```python
from build123d import *

# Parameters (mm, degrees)
SALIENTE_EXTRUIR1_DEPTH = 3


with BuildPart() as part:
    # Model → Saliente-Extruir1 (new body)
    with BuildSketch(Plane.XY):
        with BuildLine():
            Line((149.34213351, 211.823953209), (158.34213351, 211.823953209))
            Line((158.34213351, 211.823953209), (162.84213351, 211.823953209))
            Line((162.84213351, 211.823953209), (162.84213351, 198.323953209))
            Line((162.84213351, 198.323953209), (162.84213351, 193.823953209))
            Line((162.84213351, 193.823953209), (158.34213351, 193.823953209))
            ThreePointArc((158.34213351, 193.823953209), (156.620058064, 194.166495313), (155.160152994, 195.141972694))
            Line((155.160152994, 195.141972694), (146.160152994, 204.141972694))
            ThreePointArc((146.160152994, 204.141972694), (145.184675613, 205.601877763), (144.84213351, 207.323953209))
            Line((144.84213351, 207.323953209), (144.84213351, 211.823953209))
            Line((144.84213351, 211.823953209), (149.34213351, 211.823953209))
        make_face()
        with BuildLine():
            Line((156.71713351, 195.823953209), (156.71713351, 200.823953209))
            ThreePointArc((156.71713351, 200.823953209), (156.936803424, 201.354283295), (157.46713351, 201.573953209))
            Line((157.46713351, 201.573953209), (159.21713351, 201.573953209))
            ThreePointArc((159.21713351, 201.573953209), (159.747463595, 201.354283295), (159.96713351, 200.823953209))
            Line((159.96713351, 200.823953209), (159.96713351, 195.823953209))
            ThreePointArc((159.96713351, 195.823953209), (159.747463595, 195.293623123), (159.21713351, 195.073953209))
            Line((159.21713351, 195.073953209), (157.46713351, 195.073953209))
            ThreePointArc((157.46713351, 195.073953209), (156.936803424, 195.293623123), (156.71713351, 195.823953209))
        make_face(mode=Mode.SUBTRACT)
        with BuildLine():
            Line((151.84213351, 205.698953209), (146.84213351, 205.698953209))
            ThreePointArc((146.84213351, 205.698953209), (146.311803424, 205.918623123), (146.09213351, 206.448953209))
            Line((146.09213351, 206.448953209), (146.09213351, 208.198953209))
            ThreePointArc((146.09213351, 208.198953209), (146.311803424, 208.729283295), (146.84213351, 208.948953209))
            Line((146.84213351, 208.948953209), (151.84213351, 208.948953209))
            ThreePointArc((151.84213351, 208.948953209), (152.372463595, 208.729283295), (152.59213351, 208.198953209))
            Line((152.59213351, 208.198953209), (152.59213351, 206.448953209))
            ThreePointArc((152.59213351, 206.448953209), (152.372463595, 205.918623123), (151.84213351, 205.698953209))
        make_face(mode=Mode.SUBTRACT)
        with BuildLine():
            Line((160.84213351, 205.698953209), (155.84213351, 205.698953209))
            ThreePointArc((155.84213351, 205.698953209), (155.311803424, 205.918623123), (155.09213351, 206.448953209))
            Line((155.09213351, 206.448953209), (155.09213351, 208.198953209))
            ThreePointArc((155.09213351, 208.198953209), (155.311803424, 208.729283295), (155.84213351, 208.948953209))
            Line((155.84213351, 208.948953209), (160.84213351, 208.948953209))
            ThreePointArc((160.84213351, 208.948953209), (161.372463595, 208.729283295), (161.59213351, 208.198953209))
            Line((161.59213351, 208.198953209), (161.59213351, 206.448953209))
            ThreePointArc((161.59213351, 206.448953209), (161.372463595, 205.918623123), (160.84213351, 205.698953209))
        make_face(mode=Mode.SUBTRACT)
    extrude(amount=SALIENTE_EXTRUIR1_DEPTH)


solid = part.part
```
Geometry check sheet. Reference: the model listing, model coordinates, mm. A direction names the side the tool comes from. Round coordinates to 2 decimals unless told otherwise and drop trailing zeros. Loops run counter-clockwise (first coordinate to the right, second up) from the corner with the lowest first, then second, coordinate; pieces in that order, holes last. Notation, with made-up numbers: (-34, 2.25) - (-9, 2.25) arc R20 ccw to (-9, 33.25) - close; hole circle Ø11 at (54, 21.5). An arc over 180 degrees is marked (long way). Write item = value, one per line. Start each with the question number.
1. Section check A-A on x = 159. Enter the section's corners in (y, z), then the cut area to 4 significant figures.
2. Section check D-D on x = 149.25. Enter the section's corners in (y, z), then the cut area to 3 significant figures.
3. Thickness scan on line 1 (X direction, y = 208.25, z = 1.55); line 2 (Y direction, x = 158.75, z = 0.9); line 3 (X direction, y = 206, z = 2.35). Record the ranges inside material, lowest first.
4. Depth check by flat-ended pin: pin 1 (5 mm diameter, centred on x = 149, y = 196.5, fed in from +Z); pin 2 (0.9 mm diameter, centred on y = 198, z = 1, fed in from -X). Enter the tip coordinate at first touch or a pass-through.
5. Section check C-C on z = 1. Give the number of separate pieces and of enclosed holes in the cut face, then the cut area to 3 significant figures.
6. Mould release check, pull along Y, two halves, no side actions. Record for faces 3 (the face through (158, 208.949, 1)), 4 (the face through (154, 211.824, 1)), 5 (the face through (162.842, 203, 1)), 6 (the face through (146.092, 207, 1)): released by +Y, released by -Y, zero draft, split by the parting line, or undercut.
7. Set-up check for faces 1 (the face through (152.592, 207, 1)), 2 (the face through (156, 205, 0)): record each of +Z, -Z, +X, -X, +Y, -Y from which the full face is reachable in a straight line by a thin tool's end or side.
8. Section check B-B on y = 198.25. Enter the section's corners in (x, z), then the cut area to 3 significant figures.
Working result:
q1.outline = (193.82, 0) - (195.07, 0) - (195.07, 3) - (193.82, 3) - close; (201.57, 0) - (205.7, 0) - (205.7, 3) - (201.57, 3) - close; (208.95, 0) - (211.82, 0) - (211.82, 3) - (208.95, 3) - close
q1.area = 24.75 mm^2
q2.outline = (201.05, 0) - (205.7, 0) - (205.7, 3) - (201.05, 3) - close; (208.95, 0) - (211.82, 0) - (211.82, 3) - (208.95, 3) - close
q2.area = 22.6 mm^2
q3.line_1 = 144.84 to 146.09, 152.59 to 155.09, 161.59 to 162.84
q3.line_2 = 193.82 to 195.07, 201.57 to 205.7, 208.95 to 211.82
q3.line_3 = 145.04 to 146.24, 152.44 to 155.24, 161.44 to 162.84
q4.pin_1 = through
q4.pin_2 = 151.85
q5.separate_pieces = 1
q5.enclosed_holes = 3
q5.area = 194 mm^2
q6.face_3 = undercut
q6.face_4 = released by +Y
q6.face_5 = zero draft
q6.face_6 = undercut
q7.face_1 = +Z, -Z
q7.face_2 = -Z, +X, -X, +Y, -Y
q8.outline = (152.05, 0) - (156.72, 0) - (156.72, 3) - (152.05, 3) - close; (159.97, 0) - (162.84, 0) - (162.84, 3) - (159.97, 3) - close
q8.area = 22.6 mm^2
